Check sheet for the modelled part. Datum: model origin and axes. Units: mm. Give positions to 0.01 mm unless a question says otherwise; leave off trailing zeros. Write each loop counter-clockwise with the first axis right and the second up, starting at its lowest first coordinate (ties: lowest second). Pieces come first, ordered by that corner, then holes. Notation, with made-up numbers: (57.5, -26.5) -> (76.5, -26.5) arc R10 cw to (76.5, -18.5) -> close; hole circle Ø9 at (-12.5, 50.5). An arc over 180 degrees is marked (long way). Answer as a JSON object with one key per item and string values.
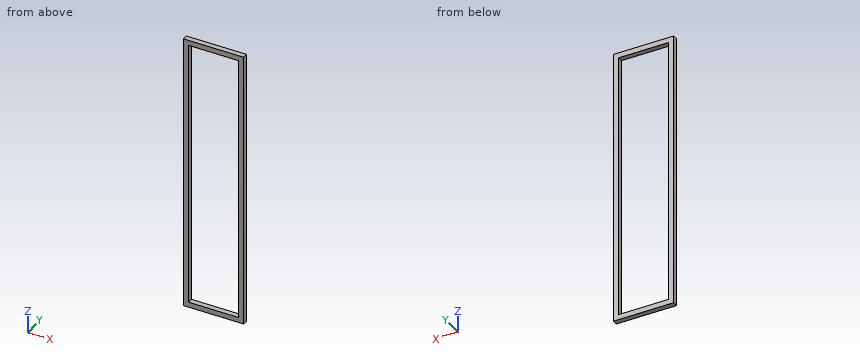
from build123d import *

# Parameters (mm, degrees)
SKETCH1_W      = 293.751
SKETCH1_H      = 1358.9
SKETCH1_W_2    = 242.951
SKETCH1_H_2    = 1308.1
EXTRUDE1_DEPTH = 25.4


with BuildPart() as part:
    # Sketch1 → Extrude1 (new body)
    with BuildSketch(Plane(origin=(0, 0, 0), x_dir=(1, 0, 0), z_dir=(0, 1, 0))):
        with Locations((76.676652699, 622.056653625)):
            Rectangle(SKETCH1_W, SKETCH1_H)
        with Locations((76.676652699, 622.056653625)):
            Rectangle(SKETCH1_W_2, SKETCH1_H_2, mode=Mode.SUBTRACT)
    extrude(amount=EXTRUDE1_DEPTH)


solid = part.part
1. Sectioned sample at C-C, the plane y = 19.75. Enter the section's corners in (x, z).
Determined:
{"outline": "(-70.2, -1301.51) -> (223.55, -1301.51) -> (223.55, 57.39) -> (-70.2, 57.39) -> close; hole (-44.8, -1276.11) -> (198.15, -1276.11) -> (198.15, 31.99) -> (-44.8, 31.99) -> close"}
2. Sectioned sample at B-B, the plane x = 115.5. Enter the section's corners in (y, z), plus the area to 3 significant figures.
Determined:
{"outline": "(0, -1301.51) -> (25.4, -1301.51) -> (25.4, -1276.11) -> (0, -1276.11) -> close; (0, 31.99) -> (25.4, 31.99) -> (25.4, 57.39) -> (0, 57.39) -> close", "area": "1,290 mm^2"}
3. Sectioned sample at A-A, the plane z = -481. Enter the section's corners in (x, y), plus the area to 3 significant figures.
Determined:
{"outline": "(-70.2, 0) -> (-44.8, 0) -> (-44.8, 25.4) -> (-70.2, 25.4) -> close; (198.15, 0) -> (223.55, 0) -> (223.55, 25.4) -> (198.15, 25.4) -> close", "area": "1,290 mm^2"}
4. Scan lines: L1, parallel to Z at x = 18.5, y = 16; L2, parallel to X at y = 1.5, z = -997. Record each from-to range of solid material in increasing order. Write a range as [from, to].
Determined:
{"L1": "[-1301.51, -1276.11], [31.99, 57.39]", "L2": "[-70.2, -44.8], [198.15, 223.55]"}
